Geometry check sheet. Reference: the model listing, model coordinates, mm. Face numbers are marked on the shaded views. Coordinates: 2 decimals unless noted, no trailing zeros. Loops run counter-clockwise (first coordinate to the right, second up) from the corner with the lowest first, then second, coordinate; pieces in that order, holes last.
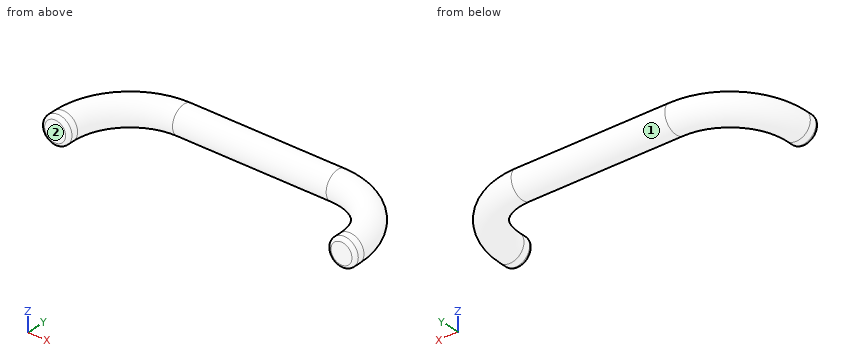
from build123d import *

# Parameters (mm, degrees)
SKETCH2_R = 4
FILLET1_R = 1


with BuildPart() as part:
    # Sweep1: sweep along a path in Sketch1
    with BuildLine(Plane.XY) as sweep1_path:
        Line((41, -22), (41, -19))
        ThreePointArc((41, -19), (35.435028843, -5.564971157), (22, 0))
        Line((22, 0), (-22, 0))
        ThreePointArc((-22, 0), (-35.435028843, -5.564971157), (-41, -19))
        Line((-41, -19), (-41, -22))
    # Sketch2 → Sweep1 (sweep)
    with BuildSketch(Plane(origin=(41, -22, 0), x_dir=(1, 0, 0), z_dir=(0, -1, 0))):
        Circle(SKETCH2_R)
    sweep(path=sweep1_path.line)

    # Fillet1
    fillet1_edges = [part.edges().sort_by_distance(p)[0] for p in [
        (37, -22, 0),
        (-37, -22, 0),
    ]]
    fillet(fillet1_edges, radius=FILLET1_R)


solid = part.part
1) Depth check by flat-ended pin: pin 1 (2 mm diameter, centred on y = -7.5, z = 1, fed in from -X); pin 2 (4 mm diameter, centred on y = -17, z = -1, fed in from +X); pin 3 (2 mm diameter, centred on x = -23.5, z = -0.5, fed in from +Y). Enter the tip coordinate at first touch or a pass-through.
Data:
pin 1: stops at x = -42.37
pin 2: stops at x = 45
pin 3: stops at y = 3.99
2) Section check A-A on z = 0. Record the cut outline in (x, y), and give its area (3 significant figures).
Data:
outline: (-45, -21) arc R1 ccw to (-44, -22) - (-38, -22) arc R1 ccw to (-37, -21) - (-37, -19) arc R15 cw to (-22, -4) - (22, -4) arc R15 cw to (37, -19) - (37, -21) arc R1 ccw to (38, -22) - (44, -22) arc R1 ccw to (45, -21) - (45, -19) arc R23 ccw to (22, 4) - (-22, 4) arc R23 ccw to (-45, -19) - close
area: 877 mm2
3) Section check C-C on x = -16.5. Record the cut outline in (y, z), and give its area (3 significant figures).
Data:
outline: circle Ø8 at (0, 0)
area: 50.3 mm2
4) Mould release check, pull along X, two halves, no side actions. Record for the marked faces 1 and 2: +X half, -X half, draft (parallel to the pull), parting line (faces both ways), or undercut.
Data:
face 1: undercut
face 2: draft
5) Section check B-B on y = -20. Record the cut outline in (x, z).
Data:
outline: circle Ø8 at (-41, 0); circle Ø8 at (41, 0)
6) Material ranges on probe 1 along X at (y, z) = (-17.25, 2.75); probe 2 along X at (y, z) = (-9.75, 0); probe 3 along Y at (x, z) = (18.5, 0.25), recorded low to high.
Data:
probe 1: x = -43.83 to -38, 38 to 43.83
probe 2: x = -43.06 to -33.81, 33.81 to 43.06
probe 3: y = -3.99 to 3.99
